```python
from build123d import *
from build123d.topology import SkipClean

# Parameters (mm, degrees)
BOSS_EXTRUDE1_DEPTH = 130
SHELL1_T            = -2.2
SKETCH3_W           = 13
SKETCH3_H           = 8.4
CUT_EXTRUDE1_DEPTH  = 2.2
SKETCH6_W           = 2.478928052
SKETCH6_H           = 13.527023683
CUT_EXTRUDE2_DEPTH  = 2.2
SKETCH4_R           = 12.5
CUT_EXTRUDE3_DEPTH  = 2.2
FILLET1_R           = 4
SKETCH7_W           = 22.6
SKETCH7_H           = 50.325296996
BOSS_EXTRUDE2_DEPTH = 3
SKETCH8_W           = 22.6
SKETCH8_H           = 23.572157484
CUT_EXTRUDE4_DEPTH  = 3
CHAMFER1_SIZE       = 10
CHAMFER1_SIZE_2     = 5.543090515
BOSS_EXTRUDE3_START = 4
BOSS_EXTRUDE3_DEPTH = 4
CUT_EXTRUDE5_DEPTH  = 5


with BuildPart() as part:
    # Sketch1 → Boss-Extrude1 (new body)
    with BuildSketch(Plane(origin=(0, 0, 0), x_dir=(1, 0, 0), z_dir=(0, 1, 0))):
        Polygon((0, 0), (41.795955874, -4.134981567), (44.45415831, 22.733847209), (2.658202436, 26.868828776), align=None)
    extrude(amount=BOSS_EXTRUDE1_DEPTH)

    # Shell1
    shell1_openings = [part.faces().sort_by_distance(p)[0] for p in [
        (22.227079155, 130, -11.366923605),
    ]]
    offset(amount=SHELL1_T, openings=shell1_openings, kind=Kind.INTERSECTION)

    # Sketch3 → Cut-Extrude1 (cut)
    with BuildSketch(Plane(origin=(41.795955874, 0, 4.134981567), x_dir=(0.09845194207530276, 0, -0.9951418065288994), z_dir=(0.9951418065288994, 0, 0.09845194207530276))):
        with Locations((13.5, 84.444630111)):
            Rectangle(SKETCH3_W, SKETCH3_H)
    extrude(amount=-CUT_EXTRUDE1_DEPTH, mode=Mode.SUBTRACT)

    # Sketch6 → Cut-Extrude2 (cut)
    with BuildSketch(Plane(origin=(41.795955874, 0, 4.134981567), x_dir=(0.09845194207530188, 0, -0.9951418065288994), z_dir=(0.9951418065288995, 0, 0.09845194207530189))):
        with Locations((23.779140081, 105.491766173)):
            Rectangle(SKETCH6_W, SKETCH6_H)
    extrude(amount=-CUT_EXTRUDE2_DEPTH, mode=Mode.SUBTRACT)

    # Sketch4 → Cut-Extrude3 (cut)
    with BuildSketch(Plane(origin=(0, 0, 0), x_dir=(0.9951418065288994, 0, 0.0984519420753021), z_dir=(-0.09845194207530208, 0, 0.9951418065288993))):
        with Locations((21, 106.537728643)):
            Circle(SKETCH4_R)
    extrude(amount=-CUT_EXTRUDE3_DEPTH, mode=Mode.SUBTRACT)

    # Fillet1
    # the kernel refuses this fillet: 4 mm, written as the material it takes off along each edge
    with BuildSketch(Plane(origin=(2.658202436, -10, -26.868828776), x_dir=(-0.0984519420753019, 0, 0.9951418065288995), z_dir=(0, 1, 0)), Plane(origin=(0, -10, 0), x_dir=(0.9951418065288994, 0, 0.09845194207530183), z_dir=(0, 1, 0))) as fillet1_piece_1:
        with BuildLine():
            CenterArc((FILLET1_R, FILLET1_R), FILLET1_R, 180, 90)
            Line((0, FILLET1_R), (0, 0))
            Line((0, 0), (FILLET1_R, 0))
        make_face()
    extrude(amount=150, mode=Mode.SUBTRACT)
    with BuildSketch(Plane(origin=(44.45415831, -10, -22.733847209), x_dir=(-0.09845194207530218, 0, 0.9951418065288994), z_dir=(0, 1, 0)), Plane(origin=(41.795955874, -10, 4.134981567), x_dir=(-0.9951418065288994, 0, -0.09845194207530182), z_dir=(0, 1, 0))) as fillet1_piece_2:
        with BuildLine():
            CenterArc((FILLET1_R, -FILLET1_R), FILLET1_R, 90, 90)
            Line((0, -FILLET1_R), (0, 0))
            Line((0, 0), (FILLET1_R, 0))
        make_face()
    extrude(amount=150, mode=Mode.SUBTRACT)

    # Sketch7 → Boss-Extrude2 (add)
    with BuildSketch(Plane(origin=(39.6066439, 0, 3.918387295), x_dir=(-0.09845194207530197, 0, 0.9951418065288994), z_dir=(-0.9951418065288995, 0, -0.09845194207530199))):
        with Locations((-13.5, 27.362648498)):
            Rectangle(SKETCH7_W, SKETCH7_H)
    extrude(amount=BOSS_EXTRUDE2_DEPTH)

    # Sketch8 → Cut-Extrude4 (cut)
    with BuildSketch(Plane(origin=(36.62121848, 0, 3.623031468), x_dir=(-0.09845194207530192, 0, 0.9951418065288994), z_dir=(-0.9951418065288995, 0, -0.09845194207530193))):
        with Locations((-13.5, 24.971356382)):
            Rectangle(SKETCH8_W, SKETCH8_H)
    extrude(amount=-CUT_EXTRUDE4_DEPTH, mode=Mode.SUBTRACT)

    # Chamfer1
    # the kernel refuses this chamfer: 10, 5.543090515 mm, written as the material it takes off along each edge
    with BuildSketch(Plane(origin=(36.837812753, 36.757435124, 1.433719494), x_dir=(-0.018642579535210594, 0.9998245108869491, -0.0018443584105231356), z_dir=(0.09845194207530193, 0, -0.9951418065288995))) as chamfer1_piece_1_section:
        Polygon((CHAMFER1_SIZE * 0.999824510887, CHAMFER1_SIZE * 0.0187335909444), (-CHAMFER1_SIZE_2 * 0.0187335909428, CHAMFER1_SIZE_2 * 0.999824510802), (0, 0), align=None)
    chamfer1_piece_1 = extrude(amount=22.6, mode=Mode.PRIVATE)
    chamfer1_piece_1 = split(chamfer1_piece_1, bisect_by=Plane(origin=(40.104235357, 40.578335675, -1.111214466), z_dir=(-0.9951418065288995, 0, -0.09845194207530193)), keep=Keep.TOP, mode=Mode.PRIVATE)
    add(chamfer1_piece_1, mode=Mode.SUBTRACT)

    # Sketch9 → Boss-Extrude3 (add)
    with BuildSketch(Plane.XZ.offset(BOSS_EXTRUDE3_START)):
        with BuildLine():
            Line((6.638769662, -26.475021008), (40.473591084, -23.127654977))
            ThreePointArc((40.473591084, -23.127654977), (43.172933538, -21.683309686), (44.060350542, -18.753279983))
            Line((44.060350542, -18.753279983), (42.189763643, 0.154414341))
            ThreePointArc((42.189763643, 0.154414341), (40.745418352, 2.853756795), (37.815388648, 3.741173799))
            Line((37.815388648, 3.741173799), (3.980567226, 0.393807768))
            ThreePointArc((3.980567226, 0.393807768), (1.281224772, -1.050537523), (0.393807768, -3.980567226))
            Line((0.393807768, -3.980567226), (2.264394668, -22.88826155))
            ThreePointArc((2.264394668, -22.88826155), (3.708739959, -25.587604004), (6.638769662, -26.475021008))
        make_face()
    extrude(amount=-BOSS_EXTRUDE3_DEPTH)

    # Sketch11 → Cut-Extrude5 (cut)
    with SkipClean():  # the faces are left unmerged after this step: merging them gives an invalid solid
        with BuildSketch(Plane.XZ.offset(4)):
            Polygon((26.115143368, -16.562744329), (28.84792956, -10.702265428), (25.13899905, -5.405363713), (21.794217599, -5.697994172), (18.449436148, -5.990624631), (15.716649956, -11.851103531), (19.425580466, -17.148005247), (22.770361917, -16.855374788), align=None)
        extrude(amount=-CUT_EXTRUDE5_DEPTH, mode=Mode.SUBTRACT)


solid = part.part
```
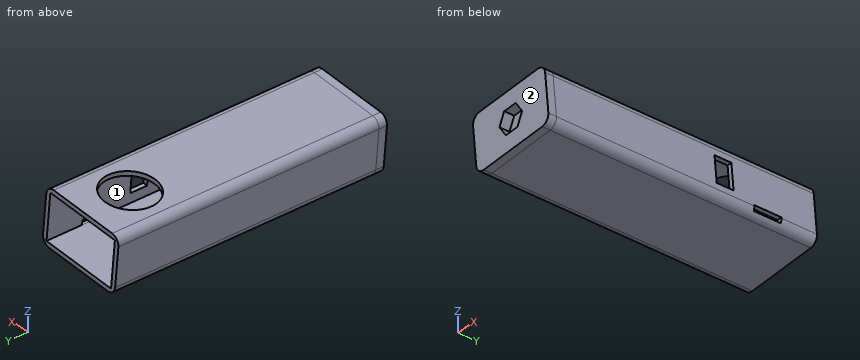
Input: part model. Units: mm. Frame: model coordinates. Face numbers are marked on the shaded views. Round coordinates to 2 decimals unless told otherwise and drop trailing zeros. Order: outer loops, then holes, each group sorted by start corner. A loop starts at its lowest first (then second) coordinate and runs counter-clockwise, first axis right, second up. Notation, with made-up numbers: (19, -4) - (42, -4) arc R17 ccw to (42, 1) - close; hole circle Ø7 at (-11, 81.5). An arc over 180 degrees is marked (long way). One line per question, with ' | ' between items. Start each with the question number.
1) Cut plane D-D, the plane z = -8. Return the cut outline in (x, y), then the cut area to 3 significant figures.
2) Contact query for flat-ended pins moving along their axis: P1, Ø6, axis at y = 75, z = -10, coming from the +X side; P2, Ø2, axis at x = 6.5, y = 70, coming from the -Z side; P3, Ø6, axis at x = 17.5, y = 94.5, coming from the +Z side; P4, Ø5, axis at y = 22, z = -14.5, coming from the -X side. Output: stop coordinate, or through.
3) Cut plane C-C, the plane y = 60.5. Return the cut outline in (x, z).
4) Ray query, probe 1 along Y at (x, z) = (17, -23); probe 2 along X at (y, z) = (16.5, -11.5); probe 3 along X at (y, z) = (100, -14). Return the intervals inside material, ascending.
5) Cut plane A-A, the plane y = 5.5. Return the cut outline in (x, z), then the cut area to 3 significant figures.
6) Pull-direction query (Z, two-part tool) for the marked faces 1 and 2; classes: +Z half, -Z half, draft (parallel to the pull), parting line (faces both ways), or undercut.
7) Cut plane B-B, the plane z = -13.5. Return the cut outline in (x, y).
Worked out:
1) outline: (0.79, -4) - (17.51, -4) - (17.51, 1) - (26.96, 1) - (26.96, -4) - (43, -4) - (43, 80.24) - (40.79, 80.24) - (40.79, 52.53) - (37.77, 52.53) - (37.77, 46.76) - (40.79, 41.35) - (40.79, 13.19) - (37.77, 13.19) - (37.77, 2.2) - (3, 2.2) - (3, 130) - (0.79, 130) - close; (40.79, 88.64) - (43, 88.64) - (43, 130) - (40.79, 130) - close | area: 820 mm^2
2) P1: stops at x = 43.49 | P2: stops at z = -26.49 | P3: stops at z = 2.02 | P4: stops at x = 1.19
3) outline: (0.39, -3.98) - (2.26, -22.89) arc R4 ccw to (6.64, -26.48) - (40.47, -23.13) arc R4 ccw to (44.06, -18.75) - (42.19, 0.15) arc R4 ccw to (37.82, 3.74) - (3.98, 0.39) arc R4 ccw to start; hole (2.41, -1.97) - (4.63, -24.46) - (42.05, -20.76) - (39.82, 1.73) - close
4) probe 1: y = -4 to 2.2 | probe 2: x = 1.14 to 3.35, 41.13 to 43.34 | probe 3: x = 1.39 to 3.6, 41.38 to 43.59
5) outline: (0.39, -3.98) - (2.26, -22.89) arc R4 ccw to (6.64, -26.48) - (40.47, -23.13) arc R4 ccw to (44.06, -18.75) - (42.19, 0.15) arc R4 ccw to (37.82, 3.74) - (3.98, 0.39) arc R4 ccw to start; hole (2.41, -1.97) - (4.63, -24.46) - (39.06, -21.06) - (36.84, 1.43) - close | area: 338 mm^2
6) face 1: undercut | face 2: draft
7) outline: (1.34, -4) - (16.87, -4) - (16.87, 1) - (27.54, 1) - (27.54, -4) - (43.54, -4) - (43.54, 80.24) - (41.33, 80.24) - (41.33, 52.53) - (38.32, 52.53) - (38.32, 46.76) - (41.33, 41.35) - (41.33, 13.19) - (38.32, 13.19) - (38.32, 2.2) - (3.55, 2.2) - (3.55, 130) - (1.34, 130) - close; (41.33, 88.64) - (43.54, 88.64) - (43.54, 130) - (41.33, 130) - close
